The model under review builds one solid part; all positions refer to its coordinate system, in mm. Coordinates: 2 decimals unless noted, no trailing zeros. Write each loop counter-clockwise with the first axis right and the second up, starting at its lowest first coordinate (ties: lowest second). Pieces come first, ordered by that corner, then holes.
1) For line 1 (X direction, y = -0.5, z = -11.25); line 2 (Y direction, x = 107, z = -0.75); line 3 (Z direction, x = 115, y = -5.5), list the stretches that pass through material, from the lowest coordinate up.
2) For P1, Ø3, axis at x = 80, z = 9.5, coming from the +Y side; P2, Ø1, axis at x = 137, y = -0.5, coming from the +Z side; P3, Ø3, axis at x = -46.5, z = -1.5, coming from the +Y side; P4, Ø3, axis at x = 272.5, z = 3, coming from the +Y side, all flat-tipped, find the tip position at first contact; note any pin that passes through.
3) Add section A-A, the plane x = -23.5. State the section outline as (y, z) points.
from build123d import *

# Parameters (mm, degrees)
BOSS_EXTRUDE1_DEPTH = 25.4


with BuildPart() as part:
    # Sketch1 → Revolve1 (revolve)
    with BuildSketch(Plane.XY):
        Polygon((369.219639575, 6.35), (369.219639575, 0), (-37.180360425, 0), (-37.180360425, 6.35), (0.919639575, 6.35), (0.919639575, 12.7), (13.619639575, 12.7), (13.619639575, 6.35), align=None)
    revolve(axis=Axis((-42.05584448, 0, 0), (1, 0, 0)))

    # Sketch2 → Boss-Extrude1 (add)
    with BuildSketch(Plane.ZY.offset(37.180360425)):
        Polygon((3.175, -5.499261314), (6.35, 0), (3.175, 5.499261314), (-3.175, 5.499261314), (-6.35, 0), (-3.175, -5.499261314), align=None)
    extrude(amount=BOSS_EXTRUDE1_DEPTH)


solid = part.part
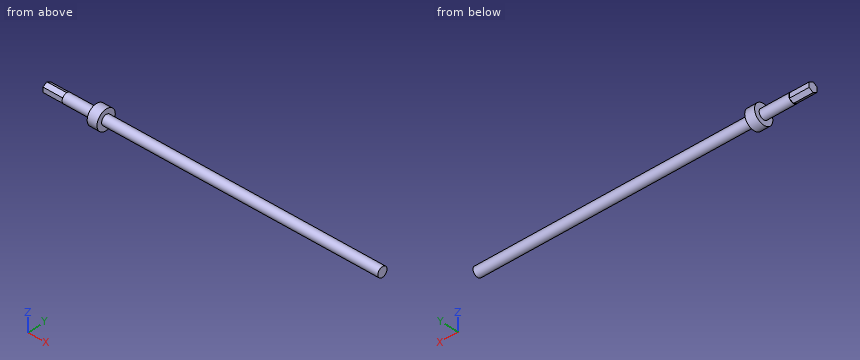
Geometry results:
1. line 1: x = 0.92 to 13.62
1. line 2: y = -6.31 to 6.31
1. line 3: z = -3.17 to 3.17
2. P1: passes through
2. P2: stops at z = 6.35
2. P3: stops at y = 5.5
2. P4: stops at y = 6.17
3. outline: circle Ø12.7 at (0, 0)
